Work out the finished part from the listing and answer in its coordinate system (mm). A direction names the side the tool comes from. Give positions to 0.01 mm unless a question says otherwise; leave off trailing zeros. Write each loop counter-clockwise with the first axis right and the second up, starting at its lowest first coordinate (ties: lowest second). Pieces come first, ordered by that corner, then holes.
1) Find section B-B (y = 30). Determine the outline of the cut face in (x, z).
2) Find section A-A (z = -5). Count the separate pieces of the cut face and the enclosed holes in it, plus the area to 3 significant figures.
3) Given pin 1 Ø4 at (x, z) = (38, 23.5) entering from +Y; pin 2 Ø4 at (x, y) = (36, -24) entering from +Z; pin 3 Ø4.5 at (y, z) = (15, 20) entering from +X, each flat-ended and moving along its own axis, determine where each tip first touches the part or whether it passes through.
4) Find section C-C (x = -50). Determine the outline of the cut face in (y, z).
5) A tool of negligible diameter and unlimited length cuts with its end or side. For faces 1 (the face through (-71, 55, 23)), 2 (the face through (-94.93, -49.73, -1.62)), from which of +Z, -Z, +X, -X, +Y, -Y can it reach the whole face along a straight path? Write none if from no direction.
6) Straight lines are drawn through the part: probe 1 along X at (y, z) = (0.5, 11.5); probe 2 along Y at (x, z) = (-92, -1); probe 3 along Y at (x, z) = (-80, 2.5). For each, find the intervals that lie inside material, in ascending order.
7) Determine the mould class of faces 3 (the face through (-93.247, -9.136, 7.146)), 4 (the face through (-84, 80, 13)), 5 (the face through (-64, 60, 35)), 6 (the face through (-12.43, 27.77, -1.62)) for opening direction Y: pulls with the +Y half, pulls with the -Y half, needs draft (parallel to the pull), parting line crosses it, or undercut.
```python
from build123d import *

# Parameters (mm, degrees)
SKETCH1_R                                       = 1.5
BOSS_EXTRUDE1_DEPTH                             = 10
BOSS_EXTRUDE2_START                             = 25
BOSS_EXTRUDE2_DEPTH                             = 25
M4_CLEARANCE_HOLE2_D                            = 4.3
CSK_FOR_M6_FLAT_HEAD_MACHINE_SCREW1_D           = 6.6
CSK_FOR_M6_FLAT_HEAD_MACHINE_SCREW1_CSINK_D     = 12.6
CSK_FOR_M6_FLAT_HEAD_MACHINE_SCREW1_CSINK_ANGLE = 90
SKETCH9_R                                       = 12.15
CUT_EXTRUDE1_DEPTH                              = 25
M3_CLEARANCE_HOLE5_D                            = 3.4
M3_CLEARANCE_HOLE5_DEPTH                        = 25


with BuildPart() as part:
    # Sketch1 → Boss-Extrude1 (new, symmetric)
    with BuildSketch(Plane.XY):
        with BuildLine():
            Line((0, 80), (-170, 80))
            Line((-170, 80), (-170, -80))
            Line((-170, -80), (0, -80))
            ThreePointArc((0, -80), (80, 0), (0, 80))
        make_face()
        with Locations((-155, 65)):
            Circle(SKETCH1_R, mode=Mode.SUBTRACT)
        with Locations((-80, 65)):
            Circle(SKETCH1_R, mode=Mode.SUBTRACT)
        with Locations((-5, 65)):
            Circle(SKETCH1_R, mode=Mode.SUBTRACT)
        with Locations(Location((-155, -65, 0), (0, 0, 180))):
            Circle(SKETCH1_R, mode=Mode.SUBTRACT)
        with Locations(Location((-80, -65, 0), (0, 0, 180))):
            Circle(SKETCH1_R, mode=Mode.SUBTRACT)
        with Locations(Location((-5, -65, 0), (0, 0, 180))):
            Circle(SKETCH1_R, mode=Mode.SUBTRACT)
        with Locations(Location((-155, 0, 0), (0, 0, 180))):
            Circle(SKETCH1_R, mode=Mode.SUBTRACT)
        with Locations((65, 0)):
            Circle(SKETCH1_R, mode=Mode.SUBTRACT)
    extrude(amount=BOSS_EXTRUDE1_DEPTH, both=True)

    # Sketch6 → Boss-Extrude2 (add)
    with BuildSketch(Plane.XY.offset(10).offset(BOSS_EXTRUDE2_START)):
        with BuildLine():
            Line((0, 80), (-170, 80))
            Line((-170, 80), (-170, -80))
            Line((-170, -80), (0, -80))
            ThreePointArc((0, -80), (80, 0), (0, 80))
        make_face()
        with BuildLine():
            Line((0, 55), (-145, 55))
            Line((-145, 55), (-145, -55))
            Line((-145, -55), (0, -55))
            ThreePointArc((0, -55), (55, 0), (0, 55))
        make_face(mode=Mode.SUBTRACT)
    extrude(amount=-BOSS_EXTRUDE2_DEPTH)

    # M4 Clearance Hole2 (through all)
    with Locations(Plane(origin=(0, 0, -10), x_dir=(1, 0, 0), z_dir=(0, 0, -1))):
        with Locations((-5, 65), (-80, 65), (-155, 65), (-155, 0), (-155, -65), (-80, -65), (-5, -65), (65, 0)):
            Hole(M4_CLEARANCE_HOLE2_D / 2)

    # CSK for M6 Flat Head Machine Screw1 (through all)
    with Locations(Plane(origin=(0, 0, 10), x_dir=(-1, 0, 0), z_dir=(0, 0, 1))):
        with Locations((92.5, -12.5), (10, -30), (110, -30), (110, 30), (10, 30), (-7.5, -47.5), (27.5, -47.5), (27.5, -12.5), (-7.5, -12.5), (-7.5, 12.5), (27.5, 12.5), (-7.5, 47.5), (27.5, 47.5), (92.5, 47.5), (92.5, 12.5), (127.5, 12.5), (127.5, 47.5), (127.5, -12.5), (127.5, -47.5), (92.5, -47.5)):
            CounterSinkHole(CSK_FOR_M6_FLAT_HEAD_MACHINE_SCREW1_D / 2, CSK_FOR_M6_FLAT_HEAD_MACHINE_SCREW1_CSINK_D / 2, counter_sink_angle=CSK_FOR_M6_FLAT_HEAD_MACHINE_SCREW1_CSINK_ANGLE)

    # Sketch9 → Cut-Extrude1 (cut)
    with BuildSketch(Plane.ZY.offset(170)):
        with Locations((20, -38)):
            Circle(SKETCH9_R)
    extrude(amount=-CUT_EXTRUDE1_DEPTH, mode=Mode.SUBTRACT)

    # M3 Clearance Hole5
    with Locations(Plane.ZY.offset(170)):
        with Locations((20, 15), (20, 40)):
            Hole(M3_CLEARANCE_HOLE5_D / 2, depth=M3_CLEARANCE_HOLE5_DEPTH)


solid = part.part
```
Results:
1. outline: (-170, -10) - (-113.3, -10) - (-113.3, 7) - (-116.3, 10) - (-145, 10) - (-145, 35) - (-170, 35) - close; (-106.7, -10) - (-13.3, -10) - (-13.3, 7) - (-16.3, 10) - (-103.7, 10) - (-106.7, 7) - close; (-6.7, -10) - (74.16, -10) - (74.16, 35) - (46.1, 35) - (46.1, 10) - (-3.7, 10) - (-6.7, 7) - close
2. separate pieces: 1
2. enclosed holes: 28
2. area: 36,500 mm2
3. pin 1: stops at y = 71.44
3. pin 2: stops at z = 10
3. pin 3: stops at x = 78.98
4. outline: (-80, -10) - (80, -10) - (80, 35) - (55, 35) - (55, 10) - (-55, 10) - (-55, 35) - (-80, 35) - close
5. face 1: +Z
5. face 2: +Z, -Z
6. probe 1: x = -170 to -157.09, -152.91 to -145, 55 to 62.91, 67.09 to 80
6. probe 2: y = -80 to -50.76, -44.24 to -15.76, -9.24 to 9.24, 15.76 to 44.24, 50.76 to 80
6. probe 3: y = -80 to -67.15, -62.85 to 62.85, 67.15 to 80
7. face 3: undercut
7. face 4: pulls with the +Y half
7. face 5: needs draft
7. face 6: undercut
